Here's how the part is built. I have some questions about the finished solid (model axes, mm). A direction names the side the tool comes from. Round coordinates to 2 decimals unless told otherwise and drop trailing zeros. Loops run counter-clockwise (first coordinate to the right, second up) from the corner with the lowest first, then second, coordinate; pieces in that order, holes last. Notation, with made-up numbers: (12, -6.5) -> (67, -6.5) arc R20 cw to (67, 12.5) -> close; hole circle Ø10 at (38, 41). An arc over 180 degrees is marked (long way). Use one line per item in the form item = value. Start each with the question number.
Item 1: I'm going to push flat-ended pins straight in: pin 1 Ø12 at (x, y) = (-16.5, 25.5) entering from -Z; pin 2 Ø8 at (y, z) = (5, 34.5) entering from +X; pin 3 Ø3 at (x, y) = (-9.5, 24) entering from -Z. Where does each tip first touch, or does it pass through?
Item 2: Thinking about a two-plate mould opening in Y: for faces 1 (the face through (20, 6, 40)), 2 (the face through (-21.606, 14.735, 35.716)), 3 (the face through (-17, 10.1, 39.5)), which applies, released by +Y, released by -Y, zero draft, split by the parting line, or undercut?
Item 3: If we section it at B-B (x = 20): Write out the boundary of the cut face in (y, z).
Item 4: For faces 4 (the face through (0, 0, 39)), 5 (the face through (-20, 10, 39)), 6 (the face through (21.81, 14.66, 35.72)), which set-ups out of +Z, -Z, +X, -X, +Y, -Y let a thin tool reach every point of the face, with its end or its side?
Item 5: If we section it at C-C (z = 12): Write out the boundary of the cut face in (x, y), then the cut area to 3 significant figures.
Item 6: If I drill on L1, parallel to Z at x = -33.5, y = 10; L2, parallel to Z at x = 30, y = 5.5; L3, parallel to X at y = 29.5, z = -3, over which ranges is the centre line in solid material (lowest first)? Write a range as [from, to].
Item 7: If we section it at A-A (y = 31): Write out the boundary of the cut face in (x, z).
Item 8: If we section it at D-D (x = -4.5): Write out the boundary of the cut face in (y, z).
```python
from build123d import *

# Parameters (mm, degrees)
F1_ANGLE = 180
F3_DEPTH = 40
F6_R     = 3
F7_DEPTH = 1


# Not quite as in the source:
# - a pattern or mirror of a feature is missing from the dataset's text; its kind, count and spacing are read off the source's solid


with BuildPart() as f1:
    # F0 (on Front) → F1 (revolve)
    with BuildSketch(Plane.XZ):
        with BuildLine():
            Line((0, 0), (0, -40))
            ThreePointArc((0, -40), (40, 0), (0, 40))
            Line((0, 40), (0, 0))
        make_face()
    revolve(axis=Axis((0, 0, 20), (0, 0, 1)), revolution_arc=F1_ANGLE)

    # F2 (on Top) → F3 (join)
    with BuildSketch(Plane.XY):
        with BuildLine():
            Line((-25, 0), (-15, 0))
            Line((-15, 0), (-15, 10))
            ThreePointArc((-15, 10), (-20, 15), (-25, 10))
            Line((-25, 10), (-25, 0))
        make_face()
        with BuildLine():
            Line((15, 10), (15, 0))
            Line((15, 0), (25, 0))
            Line((25, 0), (25, 10))
            ThreePointArc((25, 10), (20, 15), (15, 10))
        make_face()
    extrude(amount=F3_DEPTH)

    # F4 (on face) → F5 (revolve, cut)
    with BuildSketch(Plane.XZ):
        with BuildLine():
            Line((0, 38), (0, -38))
            ThreePointArc((0, -38), (38, 0), (0, 38))
        make_face()
    revolve(axis=Axis((0, 0, 0), (0, 0, 1)), mode=Mode.SUBTRACT)

    # F6 (on face) → F7 (cut)
    with BuildSketch(Plane.XY.offset(40)):
        with Locations((20, 10)):
            Circle(F6_R)
    f7 = extrude(amount=-F7_DEPTH, mode=Mode.SUBTRACT)

    # F7_copies: F7 across plane
    add(f7.mirror(Plane(origin=(0, 0, 0), x_dir=(0, 0, -1), z_dir=(-1, 0, 0))), mode=Mode.SUBTRACT)


solid = f1.part
```
Values found:
q1.pin_1 = -31.72
q1.pin_2 = 25.45
q1.pin_3 = -31.76
q2.face_1 = zero draft
q2.face_2 = released by +Y
q2.face_3 = undercut
q3.outline = (0, -34.64) arc R34.64 ccw to (15, 31.22) -> (15, 40) -> (13, 40) -> (13, 39) -> (7, 39) -> (7, 40) -> (0, 40) -> (0, 32.31) arc R32.31 cw to (0, -32.31) -> close
q4.face_4 = +Z, -Z, +X, -X, -Y
q4.face_5 = +Z
q4.face_6 = +Z, +Y
q5.outline = (-38.16, 0) -> (-36.06, 0) arc R36.06 cw to (36.06, 0) -> (38.16, 0) arc R38.16 ccw to start
q5.area = 245 mm2
q6.L1 = [-19.44, -14.89], [14.89, 19.44]
q6.L2 = [-25.88, -22.67], [22.67, 25.88]
q6.L3 = [-26.85, -23.76], [23.76, 26.85]
q7.outline = circle Ø50.56 at (0, 0); hole circle Ø43.95 at (0, 0)
q8.outline = (0, -39.75) arc R39.75 ccw to (0, 39.75) -> (0, 37.73) arc R37.73 cw to (0, -37.73) -> close
